Source: CAD feature listing. Evaluate the final solid. Frame: model axes, mm. Round coordinates to 2 decimals unless told otherwise and drop trailing zeros. Loops run counter-clockwise (first coordinate to the right, second up) from the corner with the lowest first, then second, coordinate; pieces in that order, holes last. Notation, with made-up numbers: (38.5, 57.5) - (96.5, 57.5) arc R21 ccw to (96.5, 62.5) - close; hole circle Ø7 at (-39.75, 5). An arc over 180 degrees is marked (long way). One line per question, with ' | ' between items. Start each with the question number.
1. Cut plane D-D (y = -27). Return loops of the section in (x, z).
2. Cut plane C-C (y = 0). Return loops of the section in (x, z).
3. Pin query (flat end, axial travel): pin 1 (3 mm diameter, centred on y = 6.5, z = 8, fed in from +X); pin 2 (1 mm diameter, centred on y = 40.5, z = -23.5, fed in from +X); pin 3 (4 mm diameter, centred on x = -15, z = -20, fed in from +Y). Return the tip coordinate at first contact, or that it passes through.
4. Cut plane A-A (x = 0). Return loops of the section in (y, z).
5. Mould query, pull axis Y, two halves, no side actions, for faces 1 (the flat face through (0, 62.5, 0)), 2 (the cylindrical face through (-2.226, -10.024, 0.416)), 3 (the cylindrical face through (27.447, -0.777, -11.38)). Classes: pulls with the +Y half, pulls with the -Y half, needs draft (parallel to the pull), parting line crosses it, or undercut.
6. Ray query, line 1 (Y direction, x = 0, z = -13); line 2 (Y direction, x = -7, z = -26.5); line 3 (X direction, y = 0, z = 3). Return the intervals inside material, ascending.
7. Cut plane B-B (z = 0). Return loops of the section in (x, y), then the cut area to 4 significant figures.
```python
from build123d import *

# Parameters (mm, degrees)
F0_R     = 29.713042
F1_DEPTH = 62.5
F2_R     = 10.267926
F3_DEPTH = 40
F4_R     = 7


with BuildPart() as f1:
    # F0 (on Front) → F1 (new body, symmetric)
    with BuildSketch(Plane.XZ):
        Circle(F0_R)
    extrude(amount=F1_DEPTH, both=True)

    # F2 (on Top) → F3 (cut, symmetric)
    with BuildSketch(Plane.XY):
        Circle(F2_R)
    extrude(amount=F3_DEPTH, both=True, mode=Mode.SUBTRACT)

    # F4
    f4_edges = [f1.edges().sort_by_distance(p)[0] for p in [
        (-29.713042, -62.5, 0),
        (-29.713042, 62.5, 0),
    ]]
    fillet(f4_edges, radius=F4_R)


solid = f1.part
```
Answers follow:
1) outline: circle Ø59.43 at (0, 0)
2) outline: (-10.27, -27.88) - (-10.27, 27.88) arc R29.71 ccw to start; (10.27, -27.88) arc R29.71 ccw to (10.27, 27.88) - close
3) pin 1: stops at x = 28.99 | pin 2: stops at x = 18.81 | pin 3: stops at y = 62.49
4) outline: (-62.5, -22.71) arc R7 ccw to (-55.5, -29.71) - (-10.27, -29.71) - (-10.27, 29.71) - (-55.5, 29.71) arc R7 ccw to (-62.5, 22.71) - close; (10.27, -29.71) - (55.5, -29.71) arc R7 ccw to (62.5, -22.71) - (62.5, 22.71) arc R7 ccw to (55.5, 29.71) - (10.27, 29.71) - close
5) face 1: pulls with the +Y half | face 2: undercut | face 3: needs draft
6) line 1: y = -62.5 to -10.27, 10.27 to 62.5 | line 2: y = -60.69 to -7.51, 7.51 to 60.69 | line 3: x = -29.56 to -10.27, 10.27 to 29.56
7) outline: (-29.71, -55.5) arc R7 ccw to (-22.71, -62.5) - (22.71, -62.5) arc R7 ccw to (29.71, -55.5) - (29.71, 55.5) arc R7 ccw to (22.71, 62.5) - (-22.71, 62.5) arc R7 ccw to (-29.71, 55.5) - close; hole circle Ø20.54 at (0, 0) | area: 7,055 mm2
